Geometry: final body of the model. Coordinates: model frame, mm. Give positions to 0.01 mm unless a question says otherwise; leave off trailing zeros. Write each loop counter-clockwise with the first axis right and the second up, starting at its lowest first coordinate (ties: lowest second). Pieces come first, ordered by that corner, then holes. Notation, with made-up numbers: (49, 27) - (99, 27) arc R29 ccw to (99, 65) - close; hole circle Ø3 at (5, 0). An arc over 180 degrees is marked (long way). Return JSON: item names as keys, results as strings.
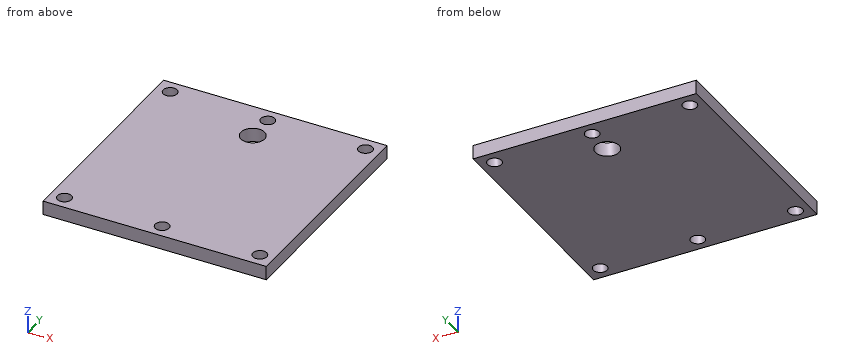
Autodesk Inventor part; units mm, degrees
ref_plane "YZ Plane" through (0, 0, 0) normal (1, 0, 0) x (0, 1, 0)
ref_plane "XZ Plane" through (0, 0, 0) normal (0, 1, 0) x (-1, 0, 0)
ref_plane "XY Plane" through (0, 0, 0) normal (0, 0, 1) x (1, 0, 0)
sketch "Sketch1" plane through (0, 0, 0) normal (0, 0, 1) x (1, 0, 0)
  line L0 (0, 0) -> (160, 0)
  line L1 (160, 0) -> (160, 160)
  line L2 (160, 160) -> (0, 160)
  line L3 (0, 160) -> (0, 0)
  line L4 (0, 160) -> (10, 160)
  dimension "d0" = 160
  dimension "d1" = 160
extrude "Extrusion1" add sketch "Sketch1" along normal blind 10
sketch "Sketch2" plane through (0, 0, 10) normal (0, 0, 1) x (1, 0, 0)
  line L0 (0, 0) -> (0, 10)
  line L1 (0, 160) -> (0, 0)
  line L2 (0, 10) -> (0, 160)
  line L3 (0, 160) -> (150, 160)
  line L4 (160, 160) -> (0, 160)
  line L5 (150, 160) -> (150, 10)
  line L6 (150, 10) -> (0, 10)
  line L7 (0, 10) -> (0, 160)
  line L8 (0, 160) -> (10, 160)
  line L9 (10, 160) -> (10, 10)
  line L10 (10, 10) -> (150, 10)
  line L11 (150, 160) -> (150, 150)
  line L12 (10, 160) -> (10, 150)
  line L13 (10, 150) -> (150, 150)
  circle A0 centre (10, 150) radius 5
  circle A1 centre (150, 150) radius 5
  circle A2 centre (10, 10) radius 5
  circle A3 centre (150, 10) radius 5
  dimension "d4" = 10
  dimension "d5" = 150
  dimension "d6" = 150
  dimension "d7" = 150
  dimension "d8" = 150
  dimension "d9" = 150
  dimension "d10" = 10
  dimension "d11" = 150
  dimension "d12" = 10
  dimension "d13" = 10
  dimension "d14" = 10
  dimension "d15" = 10
  dimension "d16" = 10
extrude "Extrusion2" cut sketch "Sketch2" against normal through all contours A2 L9 L6 | L6 A2 | A0 L13 L9 | L9 A0 | L9 A2 L6 | A1 L5 | L5 L13 A1 | L13 A0 L9 | A3 L5 L6 | L6 L5 A3 | L5 A1 L13
sketch "Sketch3" plane through (0, 0, 10) normal (0, 0, 1) x (1, 0, 0)
  line L0 (0, 160) -> (0, 0)
  line L1 (0, 0) -> (80, 0)
  line L2 (0, 0) -> (160, 0)
  line L3 (80, 0) -> (80, 10)
  line L4 (80, 10) -> (80, 150)
  circle A0 centre (80, 10) radius 5
  circle A1 centre (80, 150) radius 5
  dimension "d19" = 80
  dimension "d20" = 10
  dimension "d21" = 140
  dimension "d22" = 10
  dimension "d23" = 10
extrude "Extrusion3" cut sketch "Sketch3" against normal through all
sketch "Sketch4" plane through (0, 0, 10) normal (0, 0, 1) x (1, 0, 0)
  line L0 (160, 160) -> (0, 160)
  line L1 (0, 160) -> (80, 160)
  line L2 (80, 160) -> (80, 130)
  circle A0 centre (80, 130) radius 8.5
  point P0 (0, 0)
  dimension "d26" = 80
  dimension "d27" = 30
  dimension "d28" = 17
extrude "Extrusion4" cut sketch "Sketch4" against normal through all
properties part number "2 nd part of capping syatem"
Q1. Section query D-D, the plane x = 80. Return the cut outline in (y, z), plus the area to 3 significant figures.
Answer key:
{"outline": "(0, 0) - (5, 0) - (5, 10) - (0, 10) - close; (15, 0) - (121.5, 0) - (121.5, 10) - (15, 10) - close; (138.5, 0) - (145, 0) - (145, 10) - (138.5, 10) - close; (155, 0) - (160, 0) - (160, 10) - (155, 10) - close", "area": "1,230 mm^2"}
Q2. Section query B-B, the plane y = 150. Return the cut outline in (x, z).
Answer key:
{"outline": "(0, 0) - (5, 0) - (5, 10) - (0, 10) - close; (15, 0) - (75, 0) - (75, 10) - (15, 10) - close; (85, 0) - (145, 0) - (145, 10) - (85, 10) - close; (155, 0) - (160, 0) - (160, 10) - (155, 10) - close"}
Q3. Section query C-C, the plane z = 6.5. Return the cut outline in (x, y), plus the area to 3 significant figures.
Answer key:
{"outline": "(0, 0) - (160, 0) - (160, 160) - (0, 160) - close; hole circle Ø10 at (10, 10); hole circle Ø10 at (10, 150); hole circle Ø17 at (80, 130); hole circle Ø10 at (80, 10); hole circle Ø10 at (80, 150); hole circle Ø10 at (150, 10); hole circle Ø10 at (150, 150)", "area": "24,900 mm^2"}
Q4. Section query A-A, the plane x = 150. Return the cut outline in (y, z), plus the area to 3 significant figures.
Answer key:
{"outline": "(0, 0) - (5, 0) - (5, 10) - (0, 10) - close; (15, 0) - (145, 0) - (145, 10) - (15, 10) - close; (155, 0) - (160, 0) - (160, 10) - (155, 10) - close", "area": "1,400 mm^2"}
Q5. Material intervals for probe 1 along Y at (x, z) = (80, 7.75); probe 2 along X at (y, z) = (10, 8.25); probe 3 along X at (y, z) = (151, 9.25), sorted ascending. Write a range as [from, to].
Answer key:
{"probe 1": "y = [0, 5], [15, 121.5], [138.5, 145], [155, 160]", "probe 2": "x = [0, 5], [15, 75], [85, 145], [155, 160]", "probe 3": "x = [0, 5.1], [14.9, 75.1], [84.9, 145.1], [154.9, 160]"}
